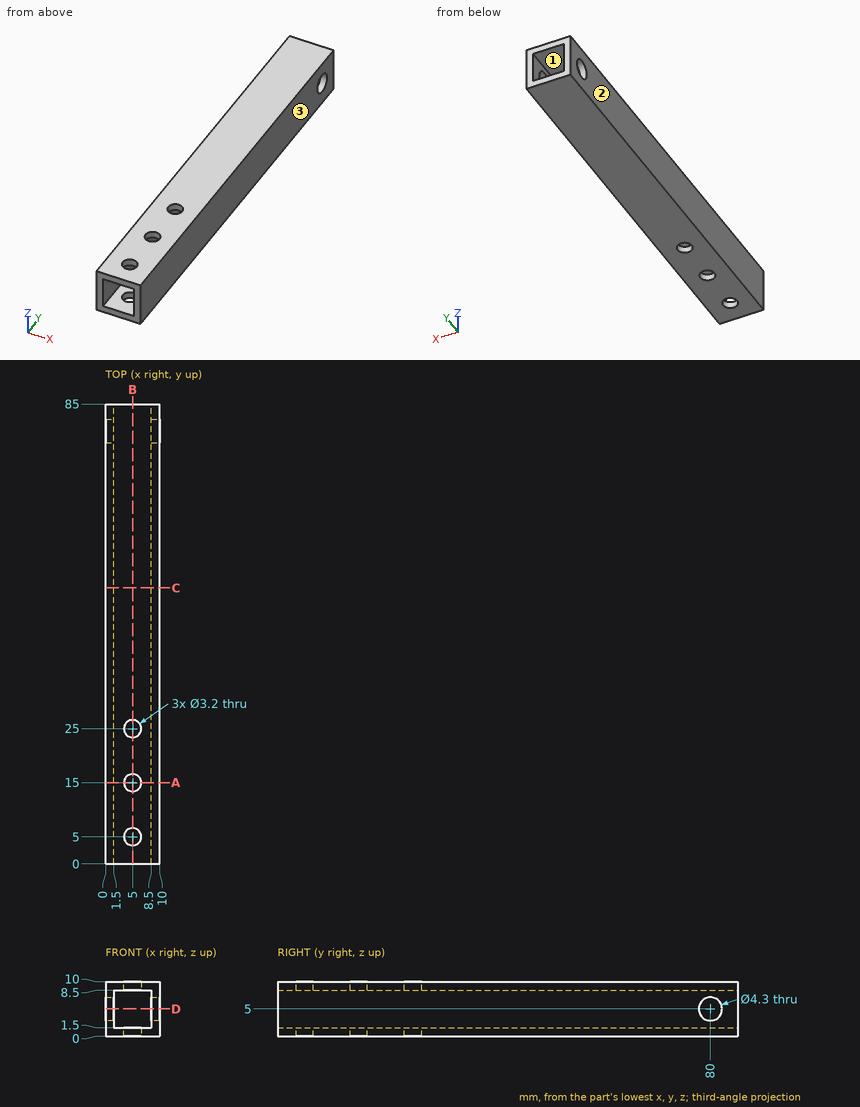
Print and shaded views of the part. All mm, measured from the part's lowest x, y and z. Coordinates: 2 decimals unless noted, no trailing zeros. Write each loop counter-clockwise with the first axis right and the second up, starting at its lowest first coordinate (ties: lowest second). Pieces come first, ordered by that corner, then holes. Notation, with made-up numbers: M 63,-24 L 98,-24 A28 ccw 98,-6 Z; hole C -11,33.25 d1. An arc over 180 degrees is marked long. Return JSON: item names as keys, results as strings.
1. Probe L1, parallel to Y at x = 5, z = 9.15; L2, parallel to Y at x = 9.45, z = 5; L3, parallel to Z at x = 8, y = 37. List the from-to ranges inside material, lowest first.
Determined:
{"L1": "0 to 3.4, 6.6 to 13.4, 16.6 to 23.4, 26.6 to 85", "L2": "0 to 77.85, 82.15 to 85", "L3": "0 to 1.5, 8.5 to 10"}
2. Saw through at B-B, the plane x = 5. Count the separate pieces of the cut face and the enclosed holes in it, then the cut area to 3 significant figures.
Determined:
{"separate pieces": "8", "enclosed holes": "0", "area": "226 mm²"}
3. Pull direction X, two halves, no side cores. Call the marked faces 1, 2 and 3: pulls with the +X half, pulls with the -X half, needs draft (parallel to the pull), parting line crosses it, or undercut.
Determined:
{"face 1": "undercut", "face 2": "pulls with the -X half", "face 3": "pulls with the +X half"}
4. Saw through at C-C, the plane y = 51. Write the cut outline in (x, z).
Determined:
{"outline": "M 0,0 L 10,0 L 10,10 L 0,10 Z; hole M 1.5,1.5 L 8.5,1.5 L 8.5,8.5 L 1.5,8.5 Z"}
5. Saw through at A-A, the plane y = 15. Write the cut outline in (x, z), then the cut area to 3 significant figures.
Determined:
{"outline": "M 0,0 L 3.4,0 L 3.4,1.5 L 1.5,1.5 L 1.5,8.5 L 3.4,8.5 L 3.4,10 L 0,10 Z; M 6.6,0 L 10,0 L 10,10 L 6.6,10 L 6.6,8.5 L 8.5,8.5 L 8.5,1.5 L 6.6,1.5 Z", "area": "41.4 mm²"}
6. Flat gauge pin, fed straight in: pin 1 Ø3.5 at (x, y) = (5.5, 29) entering from -Z. Where does the tip first touch, or does it go through?
Determined:
{"pin 1": "z = 0"}
7. Saw through at D-D, the plane z = 5. Write the cut outline in (x, y).
Determined:
{"outline": "M 0,0 L 1.5,0 L 1.5,77.85 L 0,77.85 Z; M 0,82.15 L 1.5,82.15 L 1.5,85 L 0,85 Z; M 8.5,0 L 10,0 L 10,77.85 L 8.5,77.85 Z; M 8.5,82.15 L 10,82.15 L 10,85 L 8.5,85 Z"}
